Geometry check sheet. Reference: the model listing, model coordinates, mm. Coordinates: 2 decimals unless noted, no trailing zeros. Write each loop counter-clockwise with the first axis right and the second up, starting at its lowest first coordinate (ties: lowest second). Pieces come first, ordered by that corner, then holes. Notation, with made-up numbers: (-15, 18.25) -> (14, 18.25) arc R17 cw to (14, 38.25) -> close; hole circle Ø1 at (60, 36.25). An arc over 180 degrees is marked (long way). One line per question, with ' | ' between items.
from build123d import *

# Parameters (mm, degrees)
F0_W        = 15
F0_H        = 15
F1_DEPTH    = 7
F3_DEPTH    = 10.6
F4_T1_DEPTH = 44.5


# Not quite as in the source:
# - a fillet or chamfer that OpenCascade refuses, or shapes differently, is made with other operations: its cross-section is extruded or revolved along the edge and cut away or added


with BuildPart() as f1:
    # F0 (on Top) → F1 (new body)
    with BuildSketch(Plane.XY):
        Rectangle(F0_W, F0_H)
    extrude(amount=F1_DEPTH)

    # F2 (on face) → F3 (cut)
    with BuildSketch(Plane.XZ.offset(7.5)):
        with BuildLine():
            ThreePointArc((2, 2.25), (1.9853102837, 3.5470620567), (1.5, 4.75))
            Line((1.5, 4.75), (-1.5, 4.75))
            ThreePointArc((-1.5, 4.75), (-1.9853102837, 3.5470620567), (-2, 2.25))
            Line((-2, 2.25), (2, 2.25))
        make_face()
    extrude(amount=-F3_DEPTH, mode=Mode.SUBTRACT)

    # F4: fillet of radius 7.5 on 4 edges, made by hand

    # F4_s2 → F4_t1 (cut)
    with BuildSketch(Plane.XY.offset(-18.75)):
        with BuildLine():
            ThreePointArc((0, -7.5), (-5.3033008589, -5.3033008589), (-7.5, 0))
            Line((-7.5, 0), (-7.5, -7.5))
            Line((-7.5, -7.5), (0, -7.5))
        make_face()
        with BuildLine():
            ThreePointArc((0, -7.5), (5.3033008589, -5.3033008589), (7.5, 0))
            Line((7.5, 0), (7.5, -7.5))
            Line((7.5, -7.5), (0, -7.5))
        make_face()
        with BuildLine():
            ThreePointArc((7.5, 0), (5.3033008589, 5.3033008589), (0, 7.5))
            Line((0, 7.5), (7.5, 7.5))
            Line((7.5, 7.5), (7.5, 0))
        make_face()
        with BuildLine():
            ThreePointArc((-7.5, 0), (-5.3033008589, 5.3033008589), (0, 7.5))
            Line((0, 7.5), (-7.5, 7.5))
            Line((-7.5, 7.5), (-7.5, 0))
        make_face()
    extrude(amount=F4_T1_DEPTH, mode=Mode.SUBTRACT)


solid = f1.part
1. Go/stop test with flat-tipped pins: P1, Ø0.8, axis at x = 0, z = 3, coming from the -Y side; P2, Ø3.5, axis at x = 0, y = -0.5, coming from the -Z side; P3, Ø1.5, axis at x = -1, z = 2.5, coming from the +Y side; P4, Ø1.5, axis at y = 1, z = 2.5, coming from the -X side. Record where each tip stops, or that it passes through.
Worked answers:
P1: y = 3.1 | P2: z = 0 | P3: y = 7.5 | P4: x = -7.5
2. Material ranges on line 1 (Z direction, x = 0.75, y = 2); line 2 (Y direction, x = 0.25, z = 4.25); line 3 (X direction, y = -5.75, z = 4), recorded low to high. Write a range as from..to.
Worked answers:
line 1: 0..2.25, 4.75..7 | line 2: 3.1..7.5 | line 3: -4.82..-1.86, 1.86..4.82
3. Mould release check, pull along Z, two halves, no side actions. Record for faces 1 (the face through (-1.982, -2.197, 3.565)), 2 (the face through (0, 0, 0)), 3 (the face through (0, 0, 7)): released by +Z, released by -Z, zero draft, split by the parting line, or undercut.
Worked answers:
face 1: undercut | face 2: released by -Z | face 3: released by +Z
4. Cross-section at B-B on x = -4.5. Record the boundary of the cut face in (y, z), and give its area (3 significant figures).
Worked answers:
outline: (-6, 0) -> (6, 0) -> (6, 7) -> (-6, 7) -> close | area: 84.0 mm²
5. Cross-section at D-D on y = -3.25. Record the boundary of the cut face in (x, z), and give its area (3 significant figures).
Worked answers:
outline: (-6.76, 0) -> (6.76, 0) -> (6.76, 7) -> (-6.76, 7) -> close; hole (-2, 2.25) -> (2, 2.25) arc R3.51 ccw to (1.5, 4.75) -> (-1.5, 4.75) arc R3.51 ccw to start | area: 85.1 mm²
6. Cross-section at A-A on y = 0.75. Record the boundary of the cut face in (x, z).
Worked answers:
outline: (-7.46, 0) -> (7.46, 0) -> (7.46, 7) -> (-7.46, 7) -> close; hole (-2, 2.25) -> (2, 2.25) arc R3.51 ccw to (1.5, 4.75) -> (-1.5, 4.75) arc R3.51 ccw to start
7. Cross-section at C-C on z = 1.5. Record the boundary of the cut face in (x, y).
Worked answers:
outline: circle Ø15 at (0, 0)
